Input: part model. Units: mm. Frame: model coordinates. A direction names the side the tool comes from. Coordinates: 2 decimals unless noted, no trailing zeros. Order: outer loops, then holes, each group sorted by start corner. A loop starts at its lowest first (then second) coordinate and runs counter-clockwise, first axis right, second up. Notation, with made-up numbers: (-21, -39.75) -> (-2, -39.75) arc R22 ccw to (-2, -19.75) -> close; hole circle Ø9 at (63.25, -1). An arc over 180 degrees is marked (long way). Answer as CSV lines item,"result".
from build123d import *

# Parameters (mm, degrees)
BOSS_EXTRUDE1_DEPTH     = 15
SKETCH2_R               = 13
CUT_EXTRUDE1_DEPTH      = 30
CUT_EXTRUDE2_REACH      = 53.633
SKETCH3_W               = 5
SKETCH3_H               = 14
CUT_EXTRUDE3_DEPTH      = 78.935871074
CUT_EXTRUDE3_DEPTH_BACK = 78.935871074
SKETCH4_R               = 7


with BuildPart() as part:
    # Sketch1 → Boss-Extrude1 (new, symmetric)
    with BuildSketch(Plane.XY):
        Polygon((-40, 0), (-17, 0), (-17, -5), (17, -5), (17, 0), (40, 0), (40, 6), (28, 6), (28, 30), (18, 30), (10, 35), (-10, 35), (-18, 30), (-28, 30), (-28, 6), (-40, 6), align=None)
    extrude(amount=BOSS_EXTRUDE1_DEPTH, both=True)

    # Sketch2 → Cut-Extrude1 (cut)
    with BuildSketch(Plane.XY.offset(15)):
        with Locations((0, 15.474684959)):
            Circle(SKETCH2_R)
    extrude(amount=-CUT_EXTRUDE1_DEPTH, mode=Mode.SUBTRACT)

    # Sketch3 → Cut-Extrude2 (cut, up to next)
    with BuildSketch(Plane(origin=(0, 6, 0), x_dir=(1, 0, 0), z_dir=(0, 1, 0)), mode=Mode.PRIVATE) as cut_extrude2_sk1:
        with Locations((37.5, -0.197950113)):
            Rectangle(SKETCH3_W, SKETCH3_H)
    cut_extrude2_tool1 = extrude(cut_extrude2_sk1.sketch, amount=-CUT_EXTRUDE2_REACH, mode=Mode.PRIVATE) & part.part
    cut_extrude2 = cut_extrude2_tool1.solids().sort_by_distance((37.5, 6, 0.19795))[0]
    add(cut_extrude2, mode=Mode.SUBTRACT)

    # Mirror1: Cut-Extrude2 across plane
    add(cut_extrude2.mirror(Plane(origin=(0, 0, 0), x_dir=(0, 0, 1), z_dir=(1, 0, 0))), mode=Mode.SUBTRACT)

    # Sketch4 → Cut-Extrude3 (cut, two sides: drawn at the far end of the back side and taken through both)
    with BuildSketch(Plane(origin=(28, 0, 0), x_dir=(0, 0, -1), z_dir=(1, 0, 0)).offset(-CUT_EXTRUDE3_DEPTH_BACK)):
        with Locations(Location((0, 18, 0), (0, 0, 90))):
            Circle(SKETCH4_R)
    extrude(amount=CUT_EXTRUDE3_DEPTH + CUT_EXTRUDE3_DEPTH_BACK, mode=Mode.SUBTRACT)


solid = part.part
1. Mould query, pull axis Z, two halves, no side actions, for faces 6 (the face through (0, 35, 0)), 7 (the face through (-1, 2, 15)), 8 (the face through (35, 3, 0)). Classes: released by +Z, released by -Z, zero draft, split by the parting line, or undercut.
Findings:
face 6,"zero draft"
face 7,"released by +Z"
face 8,"undercut"
2. Cut plane D-D (y = 14). Return the cut outline in (x, z), plus the area to 3 significant figures.
Findings:
outline,"(-28, -15) -> (-12.92, -15) -> (-12.92, -5.74) -> (-28, -5.74) -> close; (-28, 5.74) -> (-12.92, 5.74) -> (-12.92, 15) -> (-28, 15) -> close; (12.92, -15) -> (28, -15) -> (28, -5.74) -> (12.92, -5.74) -> close; (12.92, 5.74) -> (28, 5.74) -> (28, 15) -> (12.92, 15) -> close"
area,"558 mm2"
3. Cut plane A-A (x = 0). Return the cut outline in (y, z).
Findings:
outline,"(-5, -15) -> (2.47, -15) -> (2.47, 15) -> (-5, 15) -> close; (28.47, -15) -> (35, -15) -> (35, 15) -> (28.47, 15) -> close"
4. Cut plane C-C (y = 5). Return the cut outline in (x, z), plus the area to 3 significant figures.
Findings:
outline,"(-40, -15) -> (-7.7, -15) -> (-7.7, 15) -> (-40, 15) -> (-40, 7.2) -> (-35, 7.2) -> (-35, -6.8) -> (-40, -6.8) -> close; (7.7, -15) -> (40, -15) -> (40, -6.8) -> (35, -6.8) -> (35, 7.2) -> (40, 7.2) -> (40, 15) -> (7.7, 15) -> close"
area,"1,800 mm2"
5. Reachability of faces 1 (the face through (-33, 6, 0)), 2 (the face through (-37, 3, 7.198)), 3 (the face through (-29, 0, 0)), 4 (the face through (37, 3, 7.198)), 5 (the face through (23, 30, 0)) from +Z, -Z, +X, -X, +Y, -Y: full face, straight path, thin tool, end or side. Return the list, or none.
Findings:
face 1,"+Z, -Z, -X, +Y"
face 2,"-X, +Y, -Y"
face 3,"+Z, -Z, -X, -Y"
face 4,"+X, +Y, -Y"
face 5,"+Z, -Z, +X, +Y"
6. Ray query, line 1 along Y through (x, z) = (-19, 0); line 2 along Y through (x, z) = (0, 6); line 3 along Y through (x, z) = (34.5, -8). Return the intervals inside material, ascending.
Findings:
line 1,"y = 0 to 11, 25 to 30"
line 2,"y = -5 to 2.47, 28.47 to 35"
line 3,"y = 0 to 6"
7. Contact query for flat-ended pins moving along their axis: pin 1 (6 mm diameter, centred on x = 28, z = 11.5, fed in from +Y); pin 2 (7 mm diameter, centred on x = -32, z = 6, fed in from -Y); pin 3 (12 mm diameter, centred on y = 31, z = -9, fed in from -X); pin 4 (10 mm diameter, centred on x = 4.5, y = 14.5, fed in from +Z). Output: stop coordinate, or through.
Findings:
pin 1,"stops at y = 30"
pin 2,"stops at y = 0"
pin 3,"stops at x = -28"
pin 4,"passes through"
8. Cut plane B-B (z = 0). Return the cut outline in (x, y).
Findings:
outline,"(-35, 0) -> (-17, 0) -> (-17, -5) -> (17, -5) -> (17, 0) -> (35, 0) -> (35, 6) -> (28, 6) -> (28, 11) -> (12.21, 11) arc R13 cw to (-12.21, 11) -> (-28, 11) -> (-28, 6) -> (-35, 6) -> close; (-28, 25) -> (-8.85, 25) arc R13 cw to (8.85, 25) -> (28, 25) -> (28, 30) -> (18, 30) -> (10, 35) -> (-10, 35) -> (-18, 30) -> (-28, 30) -> close"
